Geometry: see drawing. Coordinates: mm, zero at the bounding-box minimum. A direction names the side the tool comes from. Give positions to 0.01 mm unless a question says otherwise; leave off trailing zeros. Order: outer loops, then holes, each group sorted by start corner. A loop starts at its lowest first (then second) coordinate and runs counter-clockwise, first axis right, second up. Notation, with made-up numbers: M -35,10.5 L -7,10.5 A21 ccw -7,35.5 Z; hole C -17.75,15.5 d4. An arc over 180 degrees is marked long. Answer as a JSON object with one key per item and string values. Group by question number.
1. Material intervals for L1, parallel to Y at x = 29.2, z = 15; L2, parallel to X at y = 100.5, z = 23.5, sorted ascending. Write a range as [from, to].
2. Section query B-B (x = 14.5). Output: boundary loops of the cut face in (y, z), plus the area to 3 significant figures.
3. Section query D-D (y = 118). Output: boundary loops of the cut face in (x, z).
4. Pin query (flat end, axial travel): P1, Ø15.5, axis at y = 39, z = 15, coming from the -X side. Return the tip coordinate at first contact, or that it passes through.
5. Section query C-C (y = 39). Output: boundary loops of the cut face in (x, z), plus the area to 3 significant figures.
6. Set-up query: the marked faces 1 and 2. Return all of +Z, -Z, +X, -X, +Y, -Y with unobstructed straight access to the full face (end or side cutting, diameter ignored); none if empty.
7. Section query A-A (z = 19). Output: boundary loops of the cut face in (x, y).
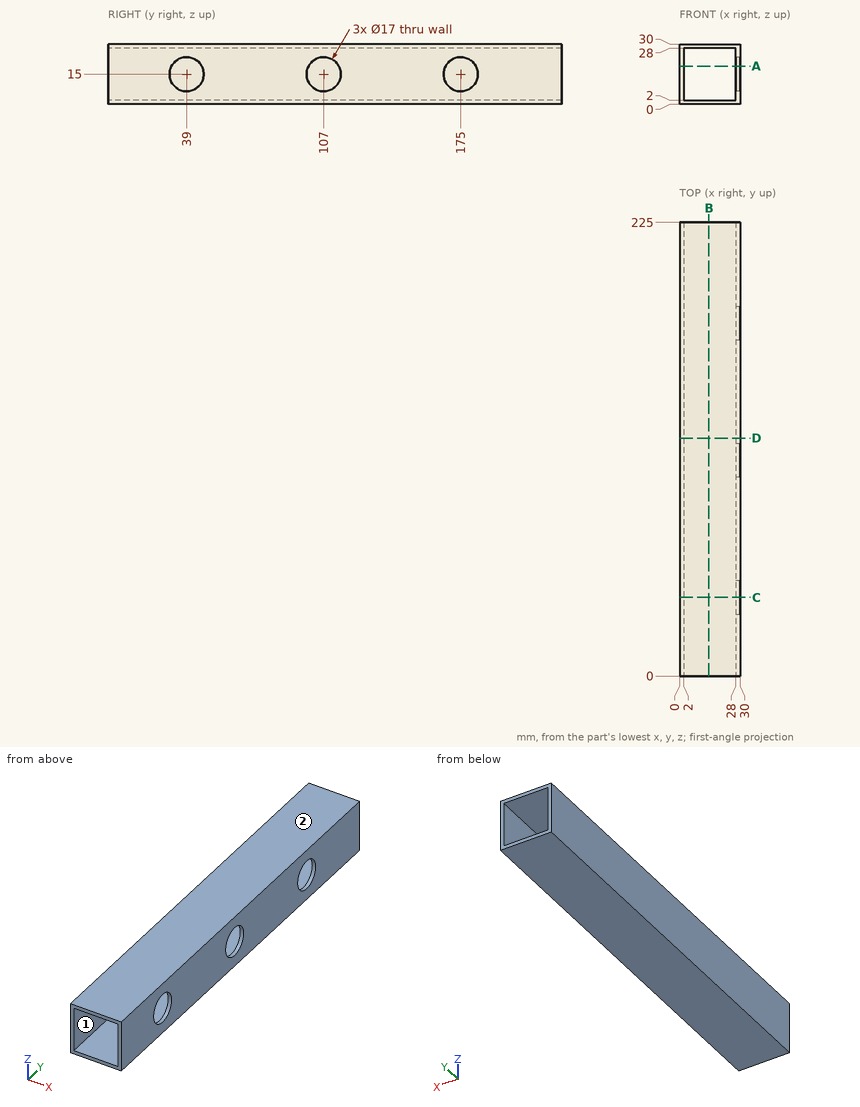
Answer sheet:
{
 "1": {"L1": "[0, 30.5], [47.5, 98.5], [115.5, 166.5], [183.5, 225]", "L2": "[0, 2], [28, 30]"},
 "2": {"outline": "M 0,0 L 225,0 L 225,2 L 0,2 Z; M 0,28 L 225,28 L 225,30 L 0,30 Z", "area": "900 mm^2"},
 "3": {"outline": "M 0,0 L 30,0 L 30,30 L 0,30 Z; hole M 2,2 L 28,2 L 28,28 L 2,28 Z"},
 "4": {"P1": "x = 0"},
 "5": {"outline": "M 0,0 L 30,0 L 30,6.5 L 28,6.5 L 28,2 L 2,2 L 2,28 L 28,28 L 28,23.5 L 30,23.5 L 30,30 L 0,30 Z", "area": "190 mm^2"},
 "6": {"face 1": "+Y, -Y", "face 2": "+Z, +X, -X, +Y, -Y"},
 "7": {"outline": "M 0,0 L 2,0 L 2,225 L 0,225 Z; M 28,0 L 30,0 L 30,31.5 L 28,31.5 Z; M 28,46.5 L 30,46.5 L 30,99.5 L 28,99.5 Z; M 28,114.5 L 30,114.5 L 30,167.5 L 28,167.5 Z; M 28,182.5 L 30,182.5 L 30,225 L 28,225 Z"}
}
